```python
from build123d import *

# Parameters (mm, degrees)
F0_R     = 3.175
F1_DEPTH = 6.35
F2_R     = 3.175
F3_DEPTH = 6.35


with BuildPart() as f1:
    # F0 (on Top) → F1 (new body, symmetric)
    with BuildSketch(Plane.XY):
        Circle(F0_R)
    extrude(amount=F1_DEPTH, both=True)

    # F2 (on Right) → F3 (join, symmetric)
    with BuildSketch(Plane.YZ):
        Circle(F2_R)
    extrude(amount=F3_DEPTH, both=True)


solid = f1.part
```
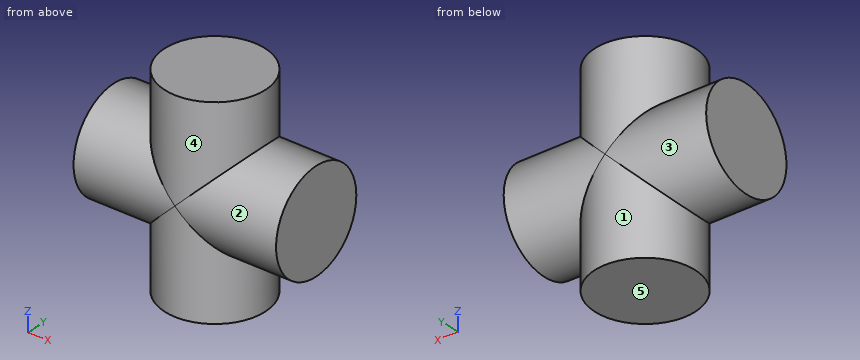
Model file for the job. Use its own axes, mm. Face numbers are marked on the shaded views. A direction names the side the tool comes from. Give positions to 0.01 mm unless a question says otherwise; leave off trailing zeros. Loops run counter-clockwise (first coordinate to the right, second up) from the corner with the lowest first, then second, coordinate; pieces in that order, holes last. Notation, with made-up numbers: (-40, 78.25) - (5, 78.25) arc R9 ccw to (5, 95.25) - close; hole circle Ø4 at (26.25, -16.5). An arc over 180 degrees is marked (long way). One line per item, written item: value. Start each with the question number.
1. Which spindle directions (+Z, -Z, +X, -X, +Y, -Y) get a long thin tool onto all of the face, cutting with end or side? Do the marked faces 1, 2, 3, 4 and 5. Say none if no direction does.
2. Probe L1, parallel to Z at x = 3.25, y = 1.5; L2, parallel to Y at x = 1, z = 5.5. List the from-to ranges inside material, lowest first. Write a range as from..to.
3. Slice it at A-A (y = 0). List the corners of the cut face in (x, z) (3 decimals), plus the area to 3 significant figures.
4. Slice it at B-B (x = 1). List the corners of the cut face in (y, z) (3 decimals), plus the area to 3 significant figures.
5. Pin check, flat tips, straight feed: pin 1 (2 mm diameter, centred on x = -1.5, z = 3, fed in from +Y); pin 2 (4 mm diameter, centred on x = -4.5, z = -0.5, fed in from -Y) (3 decimals); pin 3 (1.5 mm diameter, centred on x = 4, y = 0.5, fed in from +Z) (3 decimals). Stop position of each tip, or through.
6. Slice it at C-C (z = -4.5). List the corners of the cut face in (x, y) (3 decimals).
Solution:
1. face 1: -Z
1. face 2: +X
1. face 3: -X
1. face 4: +Z
1. face 5: -Z, +X, -X, +Y, -Y
2. L1: z = -2.8..2.8
2. L2: y = -3.01..3.01
3. outline: (-6.35, -3.175) - (-3.175, -3.175) - (-3.175, -6.35) - (3.175, -6.35) - (3.175, -3.175) - (6.35, -3.175) - (6.35, 3.175) - (3.175, 3.175) - (3.175, 6.35) - (-3.175, 6.35) - (-3.175, 3.175) - (-6.35, 3.175) - close
3. area: 121 mm^2
4. outline: (-3.013, -6.35) - (3.013, -6.35) - (3.013, -1) arc R3.175 ccw to (3.013, 1) - (3.013, 6.35) - (-3.013, 6.35) - (-3.013, 1) arc R3.175 ccw to (-3.013, -1) - close
4. area: 77.0 mm^2
5. pin 1: stops at y = 3.14
5. pin 2: stops at y = -3.175
5. pin 3: stops at z = 3.175
6. outline: circle Ø6.35 at (0, 0)
